from build123d import *

# Parameters (mm, degrees)
F0_R     = 3.3782
F0_R_2   = 2.286
F0_R_3   = 9.652
F1_DEPTH = 3.175


with BuildPart() as f1:
    # F0 (on Front) → F1 (new body)
    with BuildSketch(Plane.XZ):
        with BuildLine():
            Line((31.75, -15.634657), (31.75, 0))
            ThreePointArc((31.75, 0), (0, 31.75), (-31.75, 0))
            Line((-31.75, 0), (-31.75, -15.634657))
            Line((-31.75, -15.634657), (-31.75, -47.865343))
            Line((-31.75, -47.865343), (31.75, -47.865343))
            Line((31.75, -47.865343), (31.75, -15.634657))
        make_face()
        with Locations((-19.05, -35.438904)):
            Circle(F0_R, mode=Mode.SUBTRACT)
        with Locations((19.05, -35.438904)):
            Circle(F0_R, mode=Mode.SUBTRACT)
        with Locations((17.7292, -17.7292)):
            Circle(F0_R_2, mode=Mode.SUBTRACT)
        with Locations((-17.7292, 17.7292)):
            Circle(F0_R_2, mode=Mode.SUBTRACT)
        Circle(F0_R_3, mode=Mode.SUBTRACT)
    extrude(amount=F1_DEPTH)


solid = f1.part
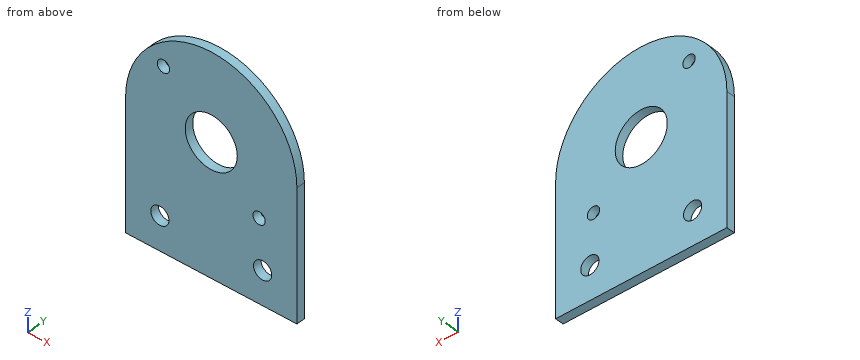
CAD build for the part. Positions are in the model's coordinates, mm. Give positions to 0.01 mm unless a question says otherwise; leave off trailing zeros. Loops run counter-clockwise (first coordinate to the right, second up) from the corner with the lowest first, then second, coordinate; pieces in that order, holes last. Notation, with made-up numbers: M -1,-1.75 L 16,-1.75 A27 cw 16,25.25 Z; hole C -38,67 d11. An arc over 180 degrees is marked long. One line per question, with ' | ' between items. Start each with the question number.
1. Saw through at B-B on z = 4. Give the cut face in (x, y) (3 decimals), plus the area to 3 significant figures.
2. Saw through at A-A on x = 0. Give the cut face in (y, z) (3 decimals), plus the area to 3 significant figures.
3. Flat gauge pins, fed straight in: pin 1 (11 mm diameter, centred on x = 19.05, z = -35.44, fed in from -Y) (3 decimals); pin 2 (17.5 mm diameter, centred on x = 0, z = 0, fed in from +Y); pin 3 (1.5 mm diameter, centred on y = -2, z = 9, fed in from -X). Where does each tip first touch, or does it go through?
4. Saw through at D-D on y = -1.5. Give the cut face in (x, z), plus the area to 3 significant figures.
5. Probe L1, parallel to Z at x = 17, y = -0.25; L2, parallel to Z at x = -16.5, y = -0.45; L3, parallel to X at y = -1.75, z = 6. List the from-to ranges inside material, lowest first. Write a range as from..to.
6. Saw through at C-C on x = -19.05. Give the cut face in (y, z) (3 decimals).
Result sheet:
1) outline: M -31.497,-3.175 L -8.784,-3.175 L -8.784,0 L -31.497,0 Z; M 8.784,-3.175 L 31.497,-3.175 L 31.497,0 L 8.784,0 Z | area: 144 mm^2
2) outline: M -3.175,-47.865 L 0,-47.865 L 0,-9.652 L -3.175,-9.652 Z; M -3.175,9.652 L 0,9.652 L 0,31.75 L -3.175,31.75 Z | area: 191 mm^2
3) pin 1: stops at y = -3.175 | pin 2: passes through | pin 3: stops at x = -30.66
4) outline: M -31.75,-47.87 L 31.75,-47.87 L 31.75,0 A31.75 ccw -31.75,0 Z; hole C -19.05,-35.44 d6.76; hole C -17.73,17.73 d4.57; hole C 0,0 d19.3; hole C 17.73,-17.73 d4.57; hole C 19.05,-35.44 d6.76 | area: 4,230 mm^2
5) L1: z = -47.87..-38.12, -32.75..-19.9, -15.56..26.82 | L2: z = -47.87..-37.65, -33.22..15.8, 19.66..27.13 | L3: x = -31.18..-7.56, 7.56..31.18
6) outline: M -3.175,-47.865 L 0,-47.865 L 0,-38.817 L -3.175,-38.817 Z; M -3.175,-32.061 L 0,-32.061 L 0,15.863 L -3.175,15.863 Z; M -3.175,19.595 L 0,19.595 L 0,25.4 L -3.175,25.4 Z
